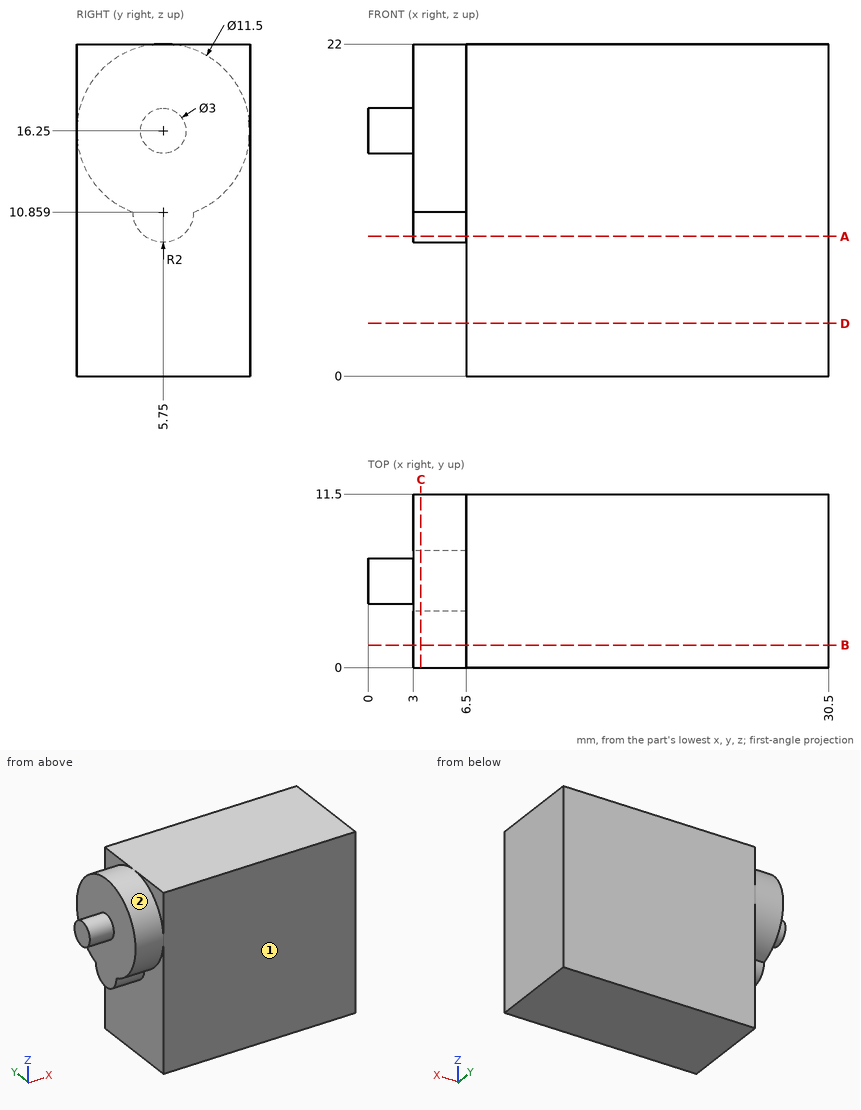
Job drawing, mm, ordinate dimensions from the low corner. One solid piece. A direction names the side the tool comes from. Coordinates: 2 decimals unless noted, no trailing zeros. Write each loop counter-clockwise with the first axis right and the second up, starting at its lowest first coordinate (ties: lowest second). Pieces come first, ordered by that corner, then holes. Notation, with made-up numbers: (19.25, 36.5) - (50.25, 36.5) arc R23 ccw to (50.25, 52.5) - close; hole circle Ø1 at (42.5, -27). An arc over 180 degrees is marked (long way). Use a Markdown table: item, result. Add a question column.
Item 1: Band-saw the part on C-C, the plane x = 3.5. Give the cut face in (y, z).
Item 2: Flat gauge pin, fed straight in: pin 1 (1.7 mm diameter, centred on y = 2, z = 20.5, fed in from -X). Where does the tip first touch, or does it go through?
Item 3: 3-axis set-ups, long thin cutter, end or side, ignore diameter. For the marked faces 1 and 2: which of +Z, -Z, +X, -X, +Y, -Y reach the whole face in a straight line?
Item 4: Band-saw the part on D-D, the plane z = 3.5. Give the cut face in (x, y).
Item 5: Band-saw the part on A-A, the plane z = 9.25. Give the cut face in (x, y), and give its area (3 significant figures).
Item 6: Band-saw the part on B-B, the plane y = 1.5. Give the cut face in (x, z).
Item 7: Drill centre lines: L1, parallel to X at y = 2.75, z = 8.5; L2, parallel to X at y = 5.75, z = 12.75; L3, parallel to Z at x = 3.5, y = 4.5. Where is each one in solid material? Low to high. Write a range as from..to.
Numbers:
| question | item | result |
|---|---|---|
| 1 | outline | (3.75, 10.86) arc R2 ccw to (7.75, 10.86) arc R5.75 ccw (long way) to start |
| 2 | pin 1 | x = 3 |
| 3 | face 1 | +Z, -Z, +X, -X, -Y |
| 3 | face 2 | -X |
| 4 | outline | (6.5, 0) - (30.5, 0) - (30.5, 11.5) - (6.5, 11.5) - close |
| 5 | outline | (3, 4.56) - (6.5, 4.56) - (6.5, 0) - (30.5, 0) - (30.5, 11.5) - (6.5, 11.5) - (6.5, 6.94) - (3, 6.94) - close |
| 5 | area | 284 mm2 |
| 6 | outline | (3, 12.38) - (6.5, 12.38) - (6.5, 0) - (30.5, 0) - (30.5, 22) - (6.5, 22) - (6.5, 20.12) - (3, 20.12) - close |
| 7 | L1 | 6.5..30.5 |
| 7 | L2 | 3..30.5 |
| 7 | L3 | 9.3..21.86 |
